from build123d import *

# Parameters (mm, degrees)
SKIZZE1_W                       = 45.72
SKIZZE1_H                       = 20.83
AUFSATZ_LINEAR_AUSTRAGEN1_DEPTH = 2
SKIZZE3_W                       = 18
SKIZZE3_H                       = 10.415
SCHNITT_LINEAR_AUSTRAGEN1_DEPTH = 10
SKIZZE7_W                       = 4.16
SKIZZE7_H                       = 4.16
AUFSATZ_LINEAR_AUSTRAGEN2_DEPTH = 8
DURCHGANGSLOCH_F_R_M21_D        = 2.2


with BuildPart() as part:
    # Skizze1 → Aufsatz-Linear austragen1 (new body)
    with BuildSketch(Plane.XY):
        Rectangle(SKIZZE1_W, SKIZZE1_H)
    extrude(amount=AUFSATZ_LINEAR_AUSTRAGEN1_DEPTH)

    # Skizze3 → Schnitt-Linear austragen1 (cut)
    with BuildSketch(Plane(origin=(0, 0, 0), x_dir=(-1, 0, 0), z_dir=(0, 0, -1))):
        with Locations((0, -5.2075)):
            Rectangle(SKIZZE3_W, SKIZZE3_H)
    extrude(amount=-SCHNITT_LINEAR_AUSTRAGEN1_DEPTH, mode=Mode.SUBTRACT)

    # Skizze7 → Aufsatz-Linear austragen2 (add)
    with BuildSketch(Plane(origin=(0, 0, 0), x_dir=(-1, 0, 0), z_dir=(0, 0, -1))):
        with Locations((20.78, 8.335)):
            Rectangle(SKIZZE7_W, SKIZZE7_H)
        with Locations((-20.78, -8.335)):
            Rectangle(SKIZZE7_W, SKIZZE7_H)
    extrude(amount=AUFSATZ_LINEAR_AUSTRAGEN2_DEPTH)

    # Durchgangsloch für M21 (through all)
    with Locations(Plane(origin=(0, 0, -8), x_dir=(-1, 0, 0), z_dir=(0, 0, -1))):
        with Locations((-20.795475973, -8.476722081), (20.7772, 8.3322)):
            Hole(DURCHGANGSLOCH_F_R_M21_D / 2)


solid = part.part
CAD build for the part. Positions are in the model's coordinates, mm. A direction names the side the tool comes from. Coordinates: 2 decimals unless noted, no trailing zeros. Write each loop counter-clockwise with the first axis right and the second up, starting at its lowest first coordinate (ties: lowest second). Pieces come first, ordered by that corner, then holes. Notation, with made-up numbers: (-36.75, -37) - (11.25, -37) arc R6 cw to (11.25, -29) - close; hole circle Ø8 at (30, 9). An arc over 180 degrees is marked (long way). Use a Markdown table: item, result. Add a question column.
Item 1: Mould opens along X. For faces 5 (the face through (21.845, -8.146, -2.93)), 6 (the face through (-21, 6.255, -4)), 7 (the face through (-22.86, 4.5, 0.4)), 8 (the face through (-9, -5, 1)) say: pulls with the +X half, pulls with the -X half, needs draft (parallel to the pull), parting line crosses it, or undercut.
Item 2: 3-axis set-ups, long thin cutter, end or side, ignore diameter. For faces 1 (the face through (21, -6.255, -4)), 2 (the face through (-18.7, 8, -4)), 3 (the face through (18.7, -8, -4)), 4 (the face through (0, 0, 1)): which of +Z, -Z, +X, -X, +Y, -Y reach the whole face in a straight line?
Item 3: Flat gauge pins, fed straight in: pin 1 (1.5 mm diameter, centred on x = -15.5, y = 1.5, fed in from -Z); pin 2 (4.5 mm diameter, centred on y = -7.5, z = -4.5, fed in from -X); pin 3 (4.5 mm diameter, centred on x = -21, z = -4.5, fed in from -Y) (3 decimals). Where does each tip first touch, or does it go through?
Item 4: Drill centre lines: L1, parallel to X at y = 8.25, z = -0.75; L2, parallel to Y at x = 19.5, z = -4.5 (3 decimals); L3, parallel to Z at x = -3.5, y = 2.5. Where is each one in solid material? Low to high. Write a range as from..to.
Item 5: Band-saw the part on D-D, the plane y = 4.5. Give the cut face in (x, z), and give its area (3 significant figures).
Item 6: Band-saw the part on A-A, the plane y = -1.75. Give the cut face in (x, z).
Item 7: Band-saw the part on B-B, the plane z = -3. Give the cut face in (x, y) (3 decimals), and give its area (3 significant figures).
Item 8: Band-saw the part on C-C, the plane z = 1. Give the cut face in (x, y) (3 decimals), and give its area (3 significant figures).
Numbers:
| question | item | result |
|---|---|---|
| 1 | face 5 | undercut |
| 1 | face 6 | needs draft |
| 1 | face 7 | pulls with the -X half |
| 1 | face 8 | undercut |
| 2 | face 1 | -Z, +X, -X, +Y |
| 2 | face 2 | -Z, +X, +Y, -Y |
| 2 | face 3 | -Z, -X, +Y, -Y |
| 2 | face 4 | +Z, -Z, -Y |
| 3 | pin 1 | z = 0 |
| 3 | pin 2 | x = 18.7 |
| 3 | pin 3 | y = 6.255 |
| 4 | L1 | -22.86..-21.87, -19.68..-18.7 |
| 4 | L2 | -10.415..-6.255 |
| 4 | L3 | 0..2 |
| 5 | outline | (-22.86, 0) - (22.86, 0) - (22.86, 2) - (-22.86, 2) - close |
| 5 | area | 91.4 mm2 |
| 6 | outline | (-22.86, 0) - (-9, 0) - (-9, 2) - (-22.86, 2) - close; (9, 0) - (22.86, 0) - (22.86, 2) - (9, 2) - close |
| 7 | outline | (-22.86, 6.255) - (-18.7, 6.255) - (-18.7, 10.415) - (-22.86, 10.415) - close; (18.7, -10.415) - (22.86, -10.415) - (22.86, -6.255) - (18.7, -6.255) - close; hole circle Ø2.2 at (-20.777, 8.332); hole circle Ø2.2 at (20.795, -8.477) |
| 7 | area | 27.0 mm2 |
| 8 | outline | (-22.86, -10.415) - (-9, -10.415) - (-9, 0) - (9, 0) - (9, -10.415) - (22.86, -10.415) - (22.86, 10.415) - (-22.86, 10.415) - close; hole circle Ø2.2 at (-20.777, 8.332); hole circle Ø2.2 at (20.795, -8.477) |
| 8 | area | 757 mm2 |
